Geometry: final body of the model. Coordinates: model frame, mm. Face numbers are marked on the shaded views. A direction names the side the tool comes from. Round coordinates to 2 decimals unless told otherwise and drop trailing zeros. Loops run counter-clockwise (first coordinate to the right, second up) from the corner with the lowest first, then second, coordinate; pieces in that order, holes last. Notation, with made-up numbers: (-20.75, 1.25) -> (30.25, 1.25) arc R19 ccw to (30.25, 28.25) -> close; hole circle Ø3 at (14, 43). An arc over 180 degrees is marked (long way). Answer in a Markdown table with one row per item.
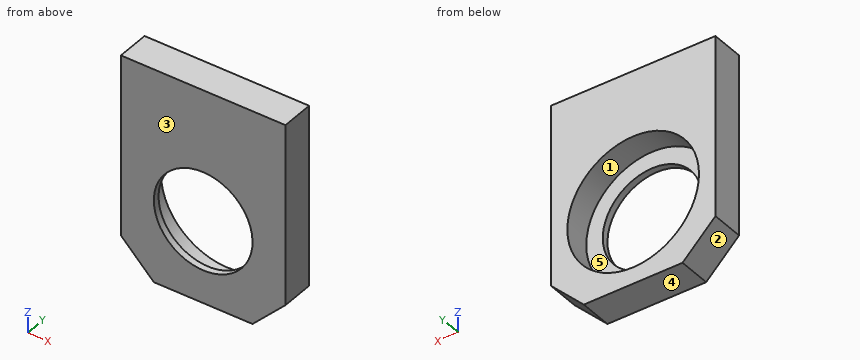
```python
from build123d import *

# Parameters (mm, degrees)
SKETCH1_W           = 41.275
SKETCH1_H           = 6.35
BOSS_EXTRUDE1_DEPTH = 15.875
SKETCH4_R           = 12.7
CUT_EXTRUDE4_DEPTH  = 5.08
SKETCH5_R           = 9.525
CUT_EXTRUDE5_DEPTH  = 6.35
CHAMFER1_SIZE       = 6.35


with BuildPart() as part:
    # Sketch1 → Boss-Extrude1 (new, symmetric)
    with BuildSketch(Plane(origin=(0, 0, 0), x_dir=(0, 0, -1), z_dir=(1, 0, 0))):
        with Locations((0, 3.175)):
            Rectangle(SKETCH1_W, SKETCH1_H)
    extrude(amount=BOSS_EXTRUDE1_DEPTH, both=True)

    # Sketch4 → Cut-Extrude4 (cut)
    with BuildSketch(Plane(origin=(0, 6.35, 0), x_dir=(1, 0, 0), z_dir=(0, 1, 0))):
        with Locations(Location((0, 4.7625, 0), (0, 0, 270))):
            Circle(SKETCH4_R)
    extrude(amount=-CUT_EXTRUDE4_DEPTH, mode=Mode.SUBTRACT)

    # Sketch5 → Cut-Extrude5 (cut)
    with BuildSketch(Plane(origin=(0, 1.27, 0), x_dir=(1, 0, 0), z_dir=(0, 1, 0))):
        with Locations(Location((0, 4.7625, 0), (0, 0, 270))):
            Circle(SKETCH5_R)
    extrude(amount=-CUT_EXTRUDE5_DEPTH, mode=Mode.SUBTRACT)

    # Chamfer1
    chamfer1_edges = [part.edges().sort_by_distance(p)[0] for p in [
        (15.875, 3.175, -20.6375),
        (-15.875, 3.175, -20.6375),
    ]]
    chamfer(chamfer1_edges, length=CHAMFER1_SIZE)


solid = part.part
```
Item 1: Line query: probe 1 along Z at (x, y) = (-0.5, 3.25); probe 2 along X at (y, z) = (3, -5) (3 decimals); probe 3 along Y at (x, z) = (12, -6.5). Output: solid intervals per line, ascending. Write a range as [from, to].
Answer:
| item | result |
|---|---|
| probe 1 | z = [-20.64, -17.45], [7.93, 20.64] |
| probe 2 | x = [-15.875, -12.698], [12.698, 15.875] |
| probe 3 | y = [0, 1.27] |
Item 2: Cut plane A-A (x = 0). Output: boundary loops of the cut face in (y, z), then the cut area to 3 significant figures.
Answer:
| item | result |
|---|---|
| outline | (0, -20.64) -> (6.35, -20.64) -> (6.35, -17.46) -> (1.27, -17.46) -> (1.27, -14.29) -> (0, -14.29) -> close; (0, 4.76) -> (1.27, 4.76) -> (1.27, 7.94) -> (6.35, 7.94) -> (6.35, 20.64) -> (0, 20.64) -> close |
| area | 109 mm² |
Item 3: Pin query (flat end, axial travel): pin 1 Ø11.5 at (x, z) = (0, -4.76) entering from +Y; pin 2 Ø12.5 at (x, z) = (1, -8.5) entering from +Y. Return the tip coordinate at first contact, or that it passes through.
Answer:
| item | result |
|---|---|
| pin 1 | passes through |
| pin 2 | stops at y = 1.27 |
Item 4: Cut plane B-B (y = 2.25). Output: boundary loops of the cut face in (x, z) (1 decimal).
Answer:
| item | result |
|---|---|
| outline | (-15.9, -14.3) -> (-9.5, -20.6) -> (9.5, -20.6) -> (15.9, -14.3) -> (15.9, 20.6) -> (-15.9, 20.6) -> close; hole circle Ø25.4 at (0, -4.8) |
Item 5: Cut plane D-D (z = -15.5). Output: boundary loops of the cut face in (x, y), then the cut area to 3 significant figures.
Answer:
| item | result |
|---|---|
| outline | (-14.66, 0) -> (14.66, 0) -> (14.66, 6.35) -> (6.78, 6.35) -> (6.78, 1.27) -> (-6.78, 1.27) -> (-6.78, 6.35) -> (-14.66, 6.35) -> close |
| area | 117 mm² |
Item 6: Cut plane C-C (z = 3.5). Output: boundary loops of the cut face in (x, y) (3 decimals), then the cut area to 3 significant figures.
Answer:
| item | result |
|---|---|
| outline | (-15.875, 0) -> (-4.739, 0) -> (-4.739, 1.27) -> (-9.645, 1.27) -> (-9.645, 6.35) -> (-15.875, 6.35) -> close; (4.739, 0) -> (15.875, 0) -> (15.875, 6.35) -> (9.645, 6.35) -> (9.645, 1.27) -> (4.739, 1.27) -> close |
| area | 91.6 mm² |
Item 7: Draft query along Z for the marked faces 3, 4 and 5. Return one class per face: pulls with the +Z half, pulls with the -Z half, needs draft (parallel to the pull), parting line crosses it, or undercut.
Answer:
| item | result |
|---|---|
| face 3 | needs draft |
| face 4 | pulls with the -Z half |
| face 5 | undercut |
Item 8: Reachability of the marked faces 1 and 2 from +Z, -Z, +X, -X, +Y, -Y: full face, straight path, thin tool, end or side. Return the list, or none.
Answer:
| item | result |
|---|---|
| face 1 | +Y |
| face 2 | -Z, -X, +Y, -Y |
